For this review, take the finished solid that the model builds, in its own axes (mm). A direction names the side the tool comes from. Coordinates: 2 decimals unless noted, no trailing zeros. Write each loop counter-clockwise with the first axis right and the second up, starting at its lowest first coordinate (ties: lowest second). Pieces come first, ordered by that corner, then holes. Notation, with made-up numbers: (27.25, 81) -> (34.25, 81) arc R32 cw to (34.25, 114) -> close; hole circle Ø4 at (68, 51.5). An arc over 180 degrees is marked (long way). Put each result on its own line as item: value. Start each with the question number.
Item 1: The part is to be moulded in two halves that separate along Y. For faces 3 (the cylindrical face through (337.337, -3.792, 0.986)), 4 (the flat face through (161, 11, 2)), 5 (the cylindrical face through (-41.385, -2.554, 0.986)), say which applies: +Y half, -Y half, draft (parallel to the pull), parting line (faces both ways), or undercut.
Item 2: To check wall thickness, follow L1, parallel to X at y = -1.5, z = 1.85; L2, parallel to Y at x = 257, z = 1.4; L3, parallel to X at y = -6, z = 1.2. State the ranges of each line that lie inside material, in increasing order.
Item 3: Consider section B-B on x = 167.5. Give the boundary of the cut face in (y, z), and give its area (3 significant figures).
Item 4: For faces 1 (the flat face through (161, 11, 0)), 2 (the flat face through (129.51, -2.01, 1.01)), list the 3-axis set-ups (+Z, -Z, +X, -X, +Y, -Y) from which the entire face can be reached by the end or side of a thin tool; tool diameter is ignored.
Item 5: Consider section C-C on z = 1.4. Give the number of separate pieces and of enclosed holes in the cut face, and give its area (3 significant figures).
Item 6: Consider section D-D on x = 123.5. Give the boundary of the cut face in (y, z).
Item 7: Insertion check: P1, Ø1, axis at x = 216, z = 1.5, coming from the +Y side; P2, Ø1, axis at x = 240, z = 1, coming from the -Y side; P3, Ø0.6, axis at y = 8, z = 0.5, coming from the -X side; P4, Ø10, axis at x = 125.5, y = -23.5, coming from the -Z side. Each pin has a flat end and moves straight along its axis. Give the tip position at first contact, or say it passes through.
Item 8: Consider section A-A on x = 250. Give the boundary of the cut face in (y, z), and give its area (3 significant figures).
```python
from build123d import *

# Parameters (mm, degrees)
SKETCH_1_R          = 9.52
EXTRUDE_1_DEPTH     = 2
SKETCH_4_W          = 43.1
SKETCH_4_H          = 0.98
SKETCH_4_W_2        = 46.2
SKETCH_4_H_2        = 8.602857229
EXTRUDE_2_DEPTH     = 2
SKETCH_2_R          = 2.05
CUT_EXTRUDE_1_DEPTH = 4
CUT_EXTRUDE_2_DEPTH = 10
FILLET_1_R          = 2
CUT_EXTRUDE_3_DEPTH = 2
FILLET_2_R          = 1.5


with BuildPart() as part:
    # 草图1 → 凸台-拉伸1 (new body)
    with BuildSketch(Plane.XY):
        with BuildLine():
            Line((328.542857143, -40.145714286), (-1.457142857, -40.145714286))
            ThreePointArc((-1.457142857, -40.145714286), (-41.457142857, -0.145714286), (-1.457142857, 39.854285714))
            Line((-1.457142857, 39.854285714), (328.542857143, 39.854285714))
            ThreePointArc((328.542857143, 39.854285714), (368.542857143, -0.145714286), (328.542857143, -40.145714286))
        make_face()
        with Locations((-1.457142857, -0.145714286)):
            Circle(SKETCH_1_R, mode=Mode.SUBTRACT)
        with Locations((328.542857143, -0.145714286)):
            Circle(SKETCH_1_R, mode=Mode.SUBTRACT)
    extrude(amount=EXTRUDE_1_DEPTH)

    # 草图4 → 凸台-拉伸2 (add)
    with BuildSketch(Plane.XY.offset(2)):
        with Locations((20.092857143, -40.635714286)):
            Rectangle(SKETCH_4_W, SKETCH_4_H)
        with Locations((18.542857143, 39.652857099)):
            Rectangle(SKETCH_4_W_2, SKETCH_4_H_2)
    extrude(amount=-EXTRUDE_2_DEPTH)

    # 草图2 → 切除-拉伸1 (cut)
    with BuildSketch(Plane.XY.offset(2)):
        with Locations((108.542857143, 33.854285714)):
            Circle(SKETCH_2_R)
        with Locations((198.542857143, 33.854285714)):
            Circle(SKETCH_2_R)
        with Locations((288.542857143, 33.854285714)):
            Circle(SKETCH_2_R)
        with Locations((108.542857143, -34.145714286)):
            Circle(SKETCH_2_R)
        with Locations((198.542857143, -34.145714286)):
            Circle(SKETCH_2_R)
        with Locations((288.542857143, -34.145714286)):
            Circle(SKETCH_2_R)
        with Locations((18.542857143, -34.145714286)):
            Circle(SKETCH_2_R)
        with Locations((18.542857143, 40.014285714)):
            Circle(SKETCH_2_R)
        Polygon((31.542857143, -21.145714286), (104.183898028, -21.145714286), (159.772133322, 20.854285714), (31.542857143, 20.854285714), align=None)
        Polygon((275.542857143, 20.854285714), (202.901816258, 20.854285714), (147.313580964, -21.145714286), (275.542857143, -21.145714286), align=None)
        Polygon((29.492857143, 41.064285714), (29.492857143, 38.964285714), (37.592857143, 38.964285714), (37.592857143, 41.064285714), (37.592857143, 53.579710622), (29.492857143, 53.579710622), align=None)
        Polygon((-0.507142857, 41.064285714), (-0.507142857, 38.964285714), (7.592857143, 38.964285714), (7.592857143, 41.064285714), (7.592857143, 53.579710622), (-0.507142857, 53.579710622), align=None)
    extrude(amount=-CUT_EXTRUDE_1_DEPTH, mode=Mode.SUBTRACT)

    # 草图3 → 切除-拉伸2 (cut)
    with BuildSketch(Plane.XY.offset(2)):
        with BuildLine():
            Line((183.145474057, 18.460683743), (135.97586329, -17.178577727))
            ThreePointArc((135.97586329, -17.178577727), (131.77376205, -16.593475022), (132.358864754, -12.391373783))
            Line((132.358864754, -12.391373783), (179.528475522, 23.247887686))
            ThreePointArc((179.528475522, 23.247887686), (183.730576762, 22.662784982), (183.145474057, 18.460683743))
        make_face()
    extrude(amount=-CUT_EXTRUDE_2_DEPTH, mode=Mode.SUBTRACT)

    # 圆角1
    fillet_1_edges = [part.edges().sort_by_distance(p)[0] for p in [
        (275.542857143, 20.854285714, 1),
        (275.542857143, -21.145714286, 1),
        (147.313580964, -21.145714286, 1),
        (202.901816258, 20.854285714, 1),
        (31.542857143, -21.145714286, 1),
        (31.542857143, 20.854285714, 1),
        (159.772133322, 20.854285714, 1),
        (104.183898028, -21.145714286, 1),
    ]]
    fillet(fillet_1_edges, radius=FILLET_1_R)

    # 草图5 → 切除-拉伸3 (cut)
    with BuildSketch(Plane.XY.offset(2)):
        with BuildLine():
            Line((20.806207352, -41.125714286), (29.507867411, -41.125714286))
            ThreePointArc((29.507867411, -41.125714286), (25.157037382, -37.88123609), (20.806207352, -41.125714286))
        make_face()
    extrude(amount=-CUT_EXTRUDE_3_DEPTH, mode=Mode.SUBTRACT)

    # 圆角2
    fillet_2_edges = [part.edges().sort_by_distance(p)[0] for p in [
        (37.592857143, 43.954285714, 1),
        (29.492857143, 43.954285714, 1),
        (-0.507142857, 43.954285714, 1),
        (7.592857143, 43.954285714, 1),
    ]]
    fillet(fillet_2_edges, radius=FILLET_2_R)


solid = part.part
```
Return value:
1. face 3: undercut
1. face 4: draft
1. face 5: parting line
2. L1: -41.43 to -10.88, 7.97 to 31.54, 130.19 to 146.77, 156.73 to 173.32, 275.54 to 319.12, 337.97 to 368.52
2. L2: -40.15 to -21.15, 20.85 to 39.85
2. L3: -41.03 to -8.96, 6.05 to 31.54, 124.23 to 140.82, 150.77 to 167.36, 275.54 to 321.04, 336.05 to 368.11
3. outline: (-40.15, 0) -> (-21.15, 0) -> (-21.15, 2) -> (-40.15, 2) -> close; (-5.89, 0) -> (6.64, 0) -> (6.64, 2) -> (-5.89, 2) -> close; (14.16, 0) -> (39.85, 0) -> (39.85, 2) -> (14.16, 2) -> close
3. area: 114 mm^2
4. face 1: -Z, +X, -X, +Y, -Y
4. face 2: +Z, -Z
5. separate pieces: 1
5. enclosed holes: 13
5. area: 22,100 mm^2
6. outline: (-40.15, 0) -> (-6.55, 0) -> (-6.55, 2) -> (-40.15, 2) -> close; (20.85, 0) -> (39.85, 0) -> (39.85, 2) -> (20.85, 2) -> close
7. P1: y = 39.85
7. P2: y = -40.15
7. P3: x = -40.68
7. P4: z = 0
8. outline: (-40.15, 0) -> (-21.15, 0) -> (-21.15, 2) -> (-40.15, 2) -> close; (20.85, 0) -> (39.85, 0) -> (39.85, 2) -> (20.85, 2) -> close
8. area: 76.0 mm^2
